```python
from build123d import *

# Parameters (mm, degrees)
F1_DEPTH    = 32
F2_R        = 5.5
F3_DEPTH    = 4
F4_R        = 1
F2_W        = 90
F2_H        = 15
F5_DEPTH    = 5
F6_T1_DEPTH = 17.9655681957
F7_SIZE2    = 2
F7_SIZE     = 5
F8_R        = 1.5
F9_R        = 6.3934301863
F9_R_2      = 6.243428201
F10_DEPTH   = 15


# Not quite as in the source:
# - a fillet or chamfer that OpenCascade refuses, or shapes differently, is made with other operations: its cross-section is extruded or revolved along the edge and cut away or added


with BuildPart() as f1:
    # F0 (on Top) → F1 (new body)
    with BuildSketch(Plane.XY):
        with BuildLine():
            ThreePointArc((0, 5), (1.4644660941, 1.4644660941), (5, 0))
            Line((5, 0), (141, 0))
            ThreePointArc((141, 0), (144.5355339059, 1.4644660941), (146, 5))
            Line((146, 5), (146, 141))
            ThreePointArc((146, 141), (144.5355339059, 144.5355339059), (141, 146))
            Line((141, 146), (5, 146))
            ThreePointArc((5, 146), (1.4644660941, 144.5355339059), (0, 141))
            Line((0, 141), (0, 5))
        make_face()
    extrude(amount=F1_DEPTH)

    # F2 (on face) → F3 (join)
    with BuildSketch(Plane.XZ):
        with Locations((107.308909297, 21.5077847242)):
            Circle(F2_R)
        with Locations((119.8735386133, 21.5077847242)):
            Circle(F2_R)
        with Locations((132.552921772, 21.5077847242)):
            Circle(F2_R)
    extrude(amount=F3_DEPTH)

    # F4
    f4_edges = [f1.edges().sort_by_distance(p)[0] for p in [
        (101.808909, -4, 21.507785),
        (114.373539, -4, 21.507785),
        (127.052922, -4, 21.507785),
    ]]
    fillet(f4_edges, radius=F4_R)

    # F2 (on face) → F5 (cut)
    with BuildSketch(Plane.XZ):
        with Locations((52.2508216836, 21.9252242893)):
            Rectangle(F2_W, F2_H)
    extrude(amount=-F5_DEPTH, mode=Mode.SUBTRACT)

    # F6: chamfer of 2 x 5 on 1 edges, made by hand

    # F6_s2 → F6_t1 (join)
    with BuildSketch(Plane.XZ.offset(-17.9655681957)):
        Polygon((12.2508216836, 29.4252242893), (7.2508216836, 27.4252242893), (7.2508216836, 29.4252242893), align=None)
    extrude(amount=F6_T1_DEPTH)

    # F7
    f7_edges = [f1.edges().sort_by_distance(p)[0] for p in [
        (97.250822, 2.5, 29.425224),
    ]]
    chamfer(f7_edges, length=F7_SIZE, length2=F7_SIZE2)

    # F8
    f8_edges = [f1.edges().sort_by_distance(p)[0] for p in [
        (92.250822, 2.5, 29.425224),
        (97.250822, 2.5, 27.425224),
        (97.250822, 2.5, 14.425224),
        (7.250822, 2.5, 14.425224),
        (7.250822, 2.5, 27.425224),
        (12.250822, 2.5, 29.425224),
    ]]
    fillet(f8_edges, radius=F8_R)

    # F9 (on face) → F10 (join)
    with BuildSketch(Plane(origin=(0, 146, 0), x_dir=(-1, 0, 0), z_dir=(0, 1, 0))):
        with Locations((-90.0897681713, 13.0425486714)):
            Circle(F9_R)
        with Locations((-69.4026425481, 13.0425486714)):
            Circle(F9_R_2)
    extrude(amount=F10_DEPTH)


solid = f1.part
```
The listing builds one solid part. Answer for the finished solid, in the listing's coordinates (mm). A direction names the side the tool comes from. Give positions to 0.01 mm unless a question says otherwise; leave off trailing zeros. Loops run counter-clockwise (first coordinate to the right, second up) from the corner with the lowest first, then second, coordinate; pieces in that order, holes last. Notation, with made-up numbers: (-28, 61.5) - (-20, 61.5) arc R9 ccw to (-20, 72.5) - close; hole circle Ø8 at (-31, -4.5). An arc over 180 degrees is marked (long way). Answer as CSV lines item,"result". Start each with the question number.
Item 1: For faces 1 (the face through (94.44, 2.47, 28.55)), 2 (the face through (107, -4, 22)), determine the directions among +Z, -Z, +X, -X, +Y, -Y from which every point of the face is accessible in a straight line to the end or side of a thin tool.
Item 2: Find the intervals of material crossed by line 1 (Y direction, x = 96.5, z = 15.5); line 2 (Y direction, x = 109, z = 9.5); line 3 (X direction, y = 148.5, z = 16), in increasing order. Write a range as from..to.
Item 3: The mould has two halves that part along X. Classify faces 3 (the face through (72, 74, 32)), 4 (the face through (84.184, 153.395, 10.594)), 5 (the face through (1, 2, 16)), 6 (the face through (114.38, -1.48, 21.75)): +X half, -X half, draft (parallel to the pull), parting line (faces both ways), or undercut.
Item 4: Each of these flat-tipped pins is pushed along its axis until it touches: pin 1 (3 mm diameter, centred on x = 115.5, z = 24, fed in from +Y); pin 2 (2.5 mm diameter, centred on y = 2, z = 19.5, fed in from -X); pin 3 (12 mm diameter, centred on x = 71, z = 21.5, fed in from -Y). Where does it stop, or does it pass through?
Item 5: A cutting plane is placed at B-B on z = 3.5. Determine the outline of the cut face in (x, y), then the cut area to 3 significant figures.
Item 6: A cutting plane is placed at A-A on x = 59. Determine the outline of the cut face in (y, z), then the cut area to 3 significant figures.
Found:
1,face 1,"-Y"
1,face 2,"+Z, -Z, +X, -X, -Y"
2,line 1,"y = 5..146"
2,line 2,"y = 0..146"
2,line 3,"x = 63.9..74.9, 84.42..95.76"
3,face 3,"draft"
3,face 4,"undercut"
3,face 5,"-X half"
3,face 6,"undercut"
4,pin 1,"stops at y = 146"
4,pin 2,"stops at x = 0.32"
4,pin 3,"stops at y = 5"
5,outline,"(0, 5) arc R5 ccw to (5, 0) - (141, 0) arc R5 ccw to (146, 5) - (146, 141) arc R5 ccw to (141, 146) - (5, 146) arc R5 ccw to (0, 141) - close"
5,area,"21,300 mm^2"
6,outline,"(0, 0) - (146, 0) - (146, 32) - (0, 32) - (0, 29.43) - (5, 29.43) - (5, 14.43) - (0, 14.43) - close"
6,area,"4,600 mm^2"
